Input: part model. Units: mm. Frame: model coordinates. A direction names the side the tool comes from. Give positions to 0.01 mm unless a question says otherwise; leave off trailing zeros. Order: outer loops, then holes, each group sorted by start corner. A loop starts at its lowest first (then second) coordinate and runs counter-clockwise, first axis right, second up. Notation, with made-up numbers: M 66,65.5 L 95,65.5 A9 cw 95,75.5 Z; hole C -34.5,18 d7. An arc over 180 degrees is marked long. Use a Markdown table: item, result.
from build123d import *

# Parameters (mm, degrees)
SKETCH1_R           = 3
BOSS_EXTRUDE1_DEPTH = 3


with BuildPart() as part:
    # Sketch1 → Boss-Extrude1 (new body)
    with BuildSketch(Plane(origin=(0, 0, 0), x_dir=(1, 0, 0), z_dir=(0, 1, 0))):
        with BuildLine():
            ThreePointArc((158.232733492, -8.975009298), (167.223082652, -3.353778756), (166.106066757, 7.190266308))
            Line((166.106066757, 7.190266308), (86.179120629, 109.260558707))
            ThreePointArc((86.179120629, 109.260558707), (78.305787364, 113.095283102), (70.432454098, 109.260558707))
            Line((70.432454098, 109.260558707), (-9.49449203, 7.190266308))
            ThreePointArc((-9.49449203, 7.190266308), (-10.611507924, -3.353778756), (-1.621158764, -8.975009298))
            Line((-1.621158764, -8.975009298), (78.305787364, -8.975009298))
            Line((78.305787364, -8.975009298), (158.232733492, -8.975009298))
        make_face()
        with Locations(Location((0, 0, 0), (0, 0, 270))):
            Circle(SKETCH1_R, mode=Mode.SUBTRACT)
        with BuildLine():
            ThreePointArc((18.910520844, 1.024990702), (9.920171683, 6.646221244), (11.037187578, 17.190266308))
            Line((11.037187578, 17.190266308), (28.959351543, 40.077672933))
            Line((28.959351543, 40.077672933), (54.70682481, 1.024990702))
            Line((54.70682481, 1.024990702), (18.910520844, 1.024990702))
        make_face(mode=Mode.SUBTRACT)
        Polygon((59.887035288, 79.573711202), (66.6846286, 79.573711202), (66.6846286, 66.364650506), (66.6846286, 19.192418643), (41.964871323, 56.686304577), align=None, mode=Mode.SUBTRACT)
        with Locations(Location((156.611574728, 0, 0), (0, 0, 270))):
            Circle(SKETCH1_R, mode=Mode.SUBTRACT)
        with BuildLine():
            Line((137.701053884, 1.024990702), (101.904749918, 1.024990702))
            Line((101.904749918, 1.024990702), (127.652223184, 40.077672933))
            Line((127.652223184, 40.077672933), (145.574387149, 17.190266308))
            ThreePointArc((145.574387149, 17.190266308), (146.691403044, 6.646221244), (137.701053884, 1.024990702))
        make_face(mode=Mode.SUBTRACT)
        Polygon((114.646703405, 56.686304577), (89.926946128, 19.192418643), (89.926946128, 79.573711202), (96.72453944, 79.573711202), align=None, mode=Mode.SUBTRACT)
        with BuildLine():
            ThreePointArc((81.284347166, 85.030073249), (80.411947198, 82.923913414), (78.305787364, 82.051513446))
            ThreePointArc((78.305787364, 82.051513446), (76.199627529, 82.923913414), (75.327227561, 85.030073249))
            Line((75.327227561, 85.030073249), (75.327227561, 102.737258658))
            ThreePointArc((75.327227561, 102.737258658), (78.126454444, 106.089918256), (81.305787364, 103.095283102))
            ThreePointArc((81.305787364, 103.095283102), (81.300422517, 102.915950182), (81.284347166, 102.737258658))
            Line((81.284347166, 102.737258658), (81.284347166, 85.030073249))
        make_face(mode=Mode.SUBTRACT)
    extrude(amount=BOSS_EXTRUDE1_DEPTH)


solid = part.part
1) Cut plane A-A on z = -31. Return loops of the section in (x, y).
Response values:
| item | result |
|---|---|
| outline | M 9.15,0 L 21.85,0 L 21.85,3 L 9.15,3 Z; M 34.94,0 L 58.9,0 L 58.9,3 L 34.94,3 Z; M 66.68,0 L 89.93,0 L 89.93,3 L 66.68,3 Z; M 97.71,0 L 121.67,0 L 121.67,3 L 97.71,3 Z; M 134.76,0 L 147.46,0 L 147.46,3 L 134.76,3 Z |
2) Cut plane C-C on y = 0.7. Return loops of the section in (x, z) (1 decimal).
Response values:
| item | result |
|---|---|
| outline | M -9.5,-7.2 L 70.4,-109.3 A10 ccw 86.2,-109.3 L 166.1,-7.2 A10 ccw 158.2,9 L -1.6,9 A10 ccw Z; hole C 0,0 d6; hole M 11,-17.2 L 29,-40.1 L 54.7,-1 L 18.9,-1 A10 ccw Z; hole M 42,-56.7 L 59.9,-79.6 L 66.7,-79.6 L 66.7,-19.2 Z; hole M 75.3,-102.7 A3 ccw long 81.3,-102.7 L 81.3,-85 A3 ccw 75.3,-85 Z; hole M 89.9,-79.6 L 96.7,-79.6 L 114.6,-56.7 L 89.9,-19.2 Z; hole M 101.9,-1 L 127.7,-40.1 L 145.6,-17.2 A10 ccw 137.7,-1 Z; hole C 156.6,0 d6 |
3) Material intervals for line 1 (X direction, y = 0.55, z = -34); line 2 (X direction, y = 2.3, z = 0); line 3 (X direction, y = 1.85, z = -53.5), sorted ascending. Write a range as from..to.
Response values:
| item | result |
|---|---|
| line 1 | x = 11.5..24.2, 32.97..56.92, 66.68..89.93, 99.69..123.65, 132.41..145.11 |
| line 2 | x = -11.57..-3, 3..153.61, 159.61..168.18 |
| line 3 | x = 26.77..44.07, 66.68..89.93, 112.55..129.84 |
4) Cut plane B-B on x = 132. Return loops of the section in (y, z) (3 decimals), and give its area (3 significant figures).
Response values:
| item | result |
|---|---|
| outline | M 0,-50.745 L 3,-50.745 L 3,-34.525 L 0,-34.525 Z; M 0,-1.025 L 3,-1.025 L 3,8.975 L 0,8.975 Z |
| area | 78.7 mm² |
5) Reachability of faces 5 (the face through (136.49, 1.48, -28.79)), 6 (the face through (167.153, 1.479, 3.494)) from +Z, -Z, +X, -X, +Y, -Y: full face, straight path, thin tool, end or side. Return the list, or none.
Response values:
| item | result |
|---|---|
| face 5 | +Y, -Y |
| face 6 | +X, +Y, -Y |
6) Mould query, pull axis X, two halves, no side actions, for faces 1 (the face through (31.03, 1.48, -58.94)), 2 (the face through (126.702, 1.479, -57.511)), 3 (the face through (9.99, 1.48, -6.51)), 4 (the face through (114.6, 1.48, -20.28)). Classes: released by +X, released by -X, zero draft, split by the parting line, or undercut.
Response values:
| item | result |
|---|---|
| face 1 | released by -X |
| face 2 | released by +X |
| face 3 | undercut |
| face 4 | undercut |
7) Cut plane D-D on z = -60.5. Return loops of the section in (x, y).
Response values:
| item | result |
|---|---|
| outline | M 32.25,0 L 44.95,0 L 44.95,3 L 32.25,3 Z; M 66.68,0 L 89.93,0 L 89.93,3 L 66.68,3 Z; M 111.66,0 L 124.36,0 L 124.36,3 L 111.66,3 Z |
8) First-contact query: pin 1 Ø1.5 at (y, z) = (1, -90) entering from +X; pin 2 Ø1.5 at (y, z) = (1, -59.5) entering from +X; pin 3 Ø1.5 at (y, z) = (2, -42.5) entering from -X. Flat tips, straight axial feed; report the tip coordinate or a pass-through.
Response values:
| item | result |
|---|---|
| pin 1 | stops at x = 101.85 |
| pin 2 | stops at x = 125.73 |
| pin 3 | stops at x = 17.57 |
